The listing builds one solid part. Answer for the finished solid, in the listing's coordinates (mm). A direction names the side the tool comes from. Coordinates: 2 decimals unless noted, no trailing zeros. Order: outer loops, then holes, each group sorted by start corner. A loop starts at its lowest first (then second) coordinate and runs counter-clockwise, first axis right, second up. Notation, with made-up numbers: (29.25, 28.5) - (70.25, 28.5) arc R25 ccw to (70.25, 42.5) - close; hole circle Ø1 at (-27, 88.25). An arc over 180 degrees is marked (long way). Use a Markdown table: item, result. Add a question column.
Item 1: Find the intervals of material crossed by line 1 along Z through (x, y) = (17, -56); line 2 along Y through (x, z) = (57, 25.5); line 3 along X through (y, z) = (24, 55), in increasing order.
Item 2: The part is cut by section D-D, the plane y = 10.5. Give the vertices of the cut face in (x, z).
Item 3: The part is cut by section A-A, the plane z = 54. Give the vertices of the cut face in (x, y), then the cut area to 3 significant figures.
Item 4: The part is cut by section C-C, the plane x = 15. Give the vertices of the cut face in (y, z), then the cut area to 3 significant figures.
Item 5: Flat-ended cylindrical pins translate along their axes: P1, Ø1, axis at x = -15.5, y = -22, coming from the +Z side; P2, Ø10, axis at x = 49.5, z = 88.5, coming from the -Y side. Find the tip coordinate at first contact, or state that the pin passes through.
Item 6: The mould has two halves that part along X. Classify faces 1 (the flat face through (84.655, 27.601, 69.368)), 2 (the cylindrical face through (4.929, 27.957, 101.384)), 3 (the flat face through (-49.177, 20, 29)): released by +X, released by -X, zero draft, split by the parting line, or undercut.
Item 7: For faces 4 (the flat face through (4, 28, 127)), 5 (the flat face through (19, 15.079, 53)), determine the directions among +Z, -Z, +X, -X, +Y, -Y from which every point of the face is accessible in a straight line to the end or side of a thin tool.
from build123d import *

# Parameters (mm, degrees)
F0_W     = 203.2
F0_H     = 101.6
F1_DEPTH = 25.4
F2_R     = 50.8
F3_W     = 177.8
F3_H     = 25.4
F4_DEPTH = 25.4
F5_DEPTH = 101.6
F6_SIZE2 = 101.59999
F6_SIZE  = 101.59999
F7_R     = 50.8
F9_D     = 50.8


# Not quite as in the source:
# - a fillet or chamfer is up to 0.001 mm smaller than in the source, because OpenCascade refuses the exact size


with BuildPart() as f1:
    # F0 (on Top) → F1 (new body)
    with BuildSketch(Plane.XY):
        with Locations((52.4225905538, -10.3211964953)):
            Rectangle(F0_W, F0_H)
    extrude(amount=F1_DEPTH)

    # F2
    f2_edges = [f1.edges().sort_by_distance(p)[0] for p in [
        (-49.177409, -61.121196, 12.7),
        (154.022591, -61.121196, 12.7),
    ]]
    fillet(f2_edges, radius=F2_R)

    # F3 (on face) → F4 (join)
    with BuildSketch(Plane.XY.offset(25.4)):
        with Locations((39.7225905538, 27.7788035047)):
            Rectangle(F3_W, F3_H)
    extrude(amount=F4_DEPTH)

    # F3 (on face) → F5 (join)
    with BuildSketch(Plane.XY.offset(25.4)):
        with Locations((39.7225905538, 27.7788035047)):
            Rectangle(F3_W, F3_H)
    extrude(amount=F5_DEPTH)

    # F6 (size 101.6 and 101.6 in the source; OpenCascade refuses exactly that, so slightly less here)
    f6_edges = [f1.edges().sort_by_distance(p)[0] for p in [
        (128.622591, 27.778804, 127),
    ]]
    chamfer(f6_edges, length=F6_SIZE, length2=F6_SIZE2)

    # F7
    f7_edges = [f1.edges().sort_by_distance(p)[0] for p in [
        (-49.177409, 27.778804, 127),
        (27.022601, 27.778804, 127),
    ]]
    fillet(f7_edges, radius=F7_R)

    # F9 (through all)
    with Locations(Plane.XZ.offset(-15.0788035047)):
        with Locations((1.6225905538, 76.2)):
            Hole(F9_D / 2)


solid = f1.part
Solution:
| question | item | result |
|---|---|---|
| 1 | line 1 | z = 0 to 25.4 |
| 1 | line 2 | y = 15.08 to 40.48 |
| 1 | line 3 | x = -49.18 to -12.37, 15.61 to 99.02 |
| 2 | outline | (-49.18, 0) - (154.02, 0) - (154.02, 25.4) - (-49.18, 25.4) - close |
| 3 | outline | (-49.18, 15.08) - (-10.72, 15.08) - (-10.72, 40.48) - (-49.18, 40.48) - close; (13.96, 15.08) - (100.02, 15.08) - (100.02, 40.48) - (13.96, 40.48) - close |
| 3 | area | 3,160 mm2 |
| 4 | outline | (-61.12, 0) - (40.48, 0) - (40.48, 54.61) - (15.08, 54.61) - (15.08, 25.4) - (-61.12, 25.4) - close; (15.08, 97.79) - (40.48, 97.79) - (40.48, 126.19) - (15.08, 126.19) - close |
| 4 | area | 4,040 mm2 |
| 5 | P1 | stops at z = 25.4 |
| 5 | P2 | stops at y = 15.08 |
| 6 | face 1 | released by +X |
| 6 | face 2 | undercut |
| 6 | face 3 | released by -X |
| 7 | face 4 | +Z, +X, -X, +Y, -Y |
| 7 | face 5 | +Z, +X, -X, -Y |
